Can you work these out from the drawing? Everything is in mm from the part's minimum corner. Give positions to 0.01 mm unless a question says otherwise; leave off trailing zeros. Write each loop counter-clockwise with the first axis right and the second up, starting at its lowest first coordinate (ties: lowest second). Pieces come first, ordered by that corner, then holes. Notation, with made-up numbers: (1, 58.25) - (28, 58.25) arc R21 cw to (28, 93.25) - close; hole circle Ø1 at (11.5, 65). An arc over 180 degrees is marked (long way). Write each question's results on one line, items separated by ' | '. Start each with the question number.
Item 1: Please list where these lines run through material, in increasing order: line 1 along X through (y, z) = (3, 4); line 2 along X through (y, z) = (12.5, 7.5).
Item 2: Suppose I cut it at B-B on y = 10. List the corners of the cut face in (x, z) for me, then the cut area to 4 significant figures.
Item 3: Will these pins go through, and if not, where does the flat tip stop? P1, Ø6, axis at y = 6.5, z = 13, coming from the +X side; P2, Ø2, axis at y = 12.5, z = 8.5, coming from the -X side; P3, Ø3, axis at y = 5.5, z = 8.5, coming from the -X side.
Item 4: Suppose I cut it at A-A on z = 6.25. List the corners of the cut face in (x, y) for me, then the cut area to 3 significant figures.
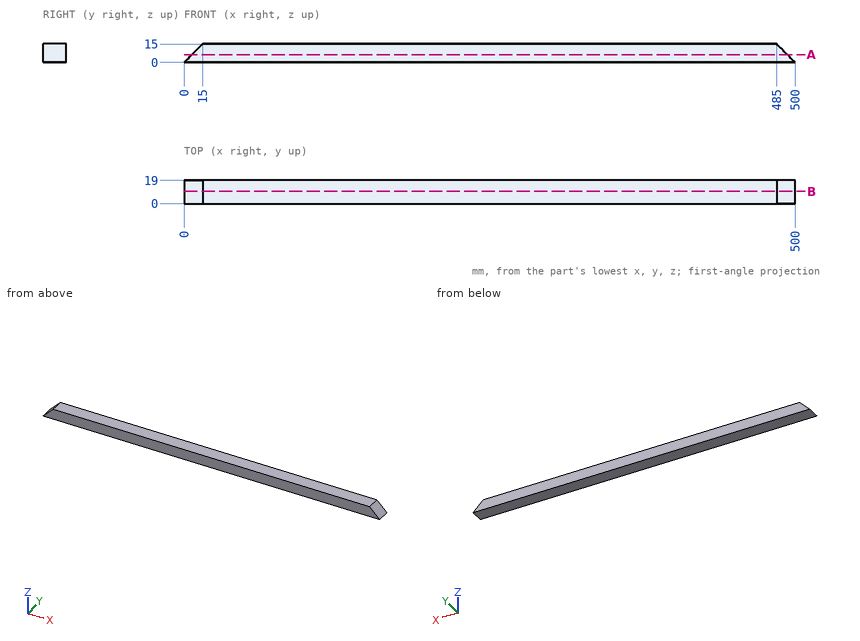
Checked values:
1) line 1: x = 4 to 496 | line 2: x = 7.5 to 492.5
2) outline: (0, 0) - (500, 0) - (485, 15) - (15, 15) - close | area: 7,275 mm^2
3) P1: stops at x = 490 | P2: stops at x = 7.5 | P3: stops at x = 7
4) outline: (6.25, 0) - (493.75, 0) - (493.75, 19) - (6.25, 19) - close | area: 9,260 mm^2
